from build123d import *

# Parameters (mm, degrees)
BOSS_EXTRUDE1_DEPTH     = 4.445
CUT_EXTRUDE2_REACH      = 37.155
CUT_EXTRUDE2_END_RADIUS = 74.075192308
SKETCH2_W               = 9.8425
SKETCH2_H               = 8.255
CUT_EXTRUDE3_REACH      = 37.155
CUT_EXTRUDE3_END_RADIUS = 74.075192308
SKETCH3_W               = 9.8425
SKETCH3_H               = 8.255
CUT_EXTRUDE5_REACH      = 37.865
CUT_EXTRUDE5_END_RADIUS = 75.345192308
SKETCH4_W               = 13.335
SKETCH4_H               = 8.255


with BuildPart() as part:
    # Sketch1 → Boss-Extrude1 (new, symmetric)
    with BuildSketch(Plane.XY):
        with BuildLine():
            Line((0, 0), (0, -3.175))
            Line((0, -3.175), (10.16, -3.175))
            Line((10.16, -3.175), (10.16, -6.35))
            Line((10.16, -6.35), (20.32, -6.35))
            Line((20.32, -6.35), (20.32, -9.525))
            Line((20.32, -9.525), (34.29, -9.525))
            Line((34.29, -9.525), (34.29, -8.255))
            ThreePointArc((34.29, -8.255), (17.634831478, -2.0928154), (0, 0))
        make_face()
    extrude(amount=BOSS_EXTRUDE1_DEPTH, both=True)

    # Cut-Extrude2: up to this cylinder (the profile starts inside it)
    cut_extrude2_end = Plane(origin=(0, -75.345192308, 0), z_dir=(0, 0, -1)) * Cylinder(CUT_EXTRUDE2_END_RADIUS, 223.460384615, mode=Mode.PRIVATE)
    # Sketch2 → Cut-Extrude2 (cut, up to the surface)
    with BuildSketch(Plane.XZ.offset(3.175), mode=Mode.PRIVATE) as cut_extrude2_sk1:
        with Locations((5.23875, 0)):
            Rectangle(SKETCH2_W, SKETCH2_H)
    cut_extrude2_tool1 = extrude(cut_extrude2_sk1.sketch, amount=-CUT_EXTRUDE2_REACH, mode=Mode.PRIVATE) & cut_extrude2_end
    add(cut_extrude2_tool1.solids().sort_by_distance((5.23875, -3.175, 0))[0], mode=Mode.SUBTRACT)

    # Cut-Extrude3: up to this cylinder (the profile starts inside it)
    cut_extrude3_end = Plane(origin=(0, -75.345192308, 0), z_dir=(0, 0, -1)) * Cylinder(CUT_EXTRUDE3_END_RADIUS, 223.460384615, mode=Mode.PRIVATE)
    # Sketch3 → Cut-Extrude3 (cut, up to the surface)
    with BuildSketch(Plane.XZ.offset(6.35), mode=Mode.PRIVATE) as cut_extrude3_sk1:
        with Locations((15.39875, 0)):
            Rectangle(SKETCH3_W, SKETCH3_H)
    cut_extrude3_tool1 = extrude(cut_extrude3_sk1.sketch, amount=-CUT_EXTRUDE3_REACH, mode=Mode.PRIVATE) & cut_extrude3_end
    add(cut_extrude3_tool1.solids().sort_by_distance((15.39875, -6.35, 0))[0], mode=Mode.SUBTRACT)

    # Cut-Extrude5: up to this cylinder (the profile starts inside it)
    cut_extrude5_end = Plane(origin=(0, -76.615192308, 0), z_dir=(0, 0, -1)) * Cylinder(CUT_EXTRUDE5_END_RADIUS, 227.420384615, mode=Mode.PRIVATE)
    # Sketch4 → Cut-Extrude5 (cut, up to the surface)
    with BuildSketch(Plane.XZ.offset(9.525), mode=Mode.PRIVATE) as cut_extrude5_sk1:
        with Locations((27.305, 0)):
            Rectangle(SKETCH4_W, SKETCH4_H)
    cut_extrude5_tool1 = extrude(cut_extrude5_sk1.sketch, amount=-CUT_EXTRUDE5_REACH, mode=Mode.PRIVATE) & cut_extrude5_end
    add(cut_extrude5_tool1.solids().sort_by_distance((27.305, -9.525, 0))[0], mode=Mode.SUBTRACT)


solid = part.part
The listing builds one solid part. Answer for the finished solid, in the listing's coordinates (mm). A direction names the side the tool comes from. Coordinates: 2 decimals unless noted, no trailing zeros. Loops run counter-clockwise (first coordinate to the right, second up) from the corner with the lowest first, then second, coordinate; pieces in that order, holes last. Notation, with made-up numbers: (11, 58) -> (38, 58) arc R20 ccw to (38, 80) -> close; hole circle Ø3 at (54.25, 26.25). An arc over 180 degrees is marked (long way). Answer in a Markdown table with one row per item. Add a question column.
1. The part is cut by section A-A, the plane y = -3.5. Write down the section's boundary in (x, z) (1 decimal).
2. For faces 1 (the flat face through (26, -7, -4.128)), 2 (the cylindrical face through (17.877, -2.152, 0.062)), 3 (the flat face through (0.16, -3.175, 0.02)), determine the directions among +Z, -Z, +X, -X, +Y, -Y from which every point of the face is accessible in a straight line to the end or side of a thin tool.
3. Consider line 1 (Z direction, x = 27, y = -7.5) (1 decimal); line 2 (X direction, y = -8.5, z = -0.5); line 3 (X direction, y = -9, z = -4). Determine where each line is inside the solid, lowest interval first. Write a range as [from, to].
4. Determine the mould class of faces 4 (the flat face through (10.478, -4, 0)), 5 (the flat face through (17, -5, 4.445)), 6 (the flat face through (34.29, -9, 0)) for opening direction Z: +Z half, -Z half, draft (parallel to the pull), parting line (faces both ways), or undercut.
5. The part is cut by section D-D, the plane y = -7.75. Write down the section's boundary in (x, z) (1 decimal), then the cut area to 3 significant figures.
6. Flat-ended cylindrical pins translate along their axes: P1, Ø1.3, axis at y = -5, z = 1, coming from the +X side; P2, Ø2.5, axis at y = -7.5, z = -0.5, coming from the +X side; P3, Ø1.5, axis at x = 9, z = 2, coming from the +Y side; P4, Ø2.5, axis at y = -7, z = 0.5, coming from the -X side. Find the tip coordinate at first contact, or state that the pin passes through.
Answer below:
| question | item | result |
|---|---|---|
| 1 | outline | (10.2, -4.4) -> (22.7, -4.4) -> (22.7, 4.4) -> (10.2, 4.4) -> close; hole (10.5, -4.1) -> (18, -4.1) -> (18, 4.1) -> (10.5, 4.1) -> close |
| 2 | face 1 | -Y |
| 2 | face 2 | +Z, -Z, +X, +Y |
| 2 | face 3 | +Z, -Z, -X, -Y |
| 3 | line 1 | [-4.4, -4.1], [4.1, 4.4] |
| 3 | line 2 | [20.32, 20.64], [32.21, 34.29] |
| 3 | line 3 | [20.32, 20.64], [33.24, 34.29] |
| 4 | face 4 | undercut |
| 4 | face 5 | +Z half |
| 4 | face 6 | draft |
| 5 | outline | (20.3, -4.4) -> (33.3, -4.4) -> (33.3, 4.4) -> (20.3, 4.4) -> close; hole (20.6, -4.1) -> (30.6, -4.1) -> (30.6, 4.1) -> (20.6, 4.1) -> close |
| 5 | area | 33.3 mm2 |
| 6 | P1 | x = 28.63 |
| 6 | P2 | x = 34.29 |
| 6 | P3 | y = -0.45 |
| 6 | P4 | x = 10.16 |
